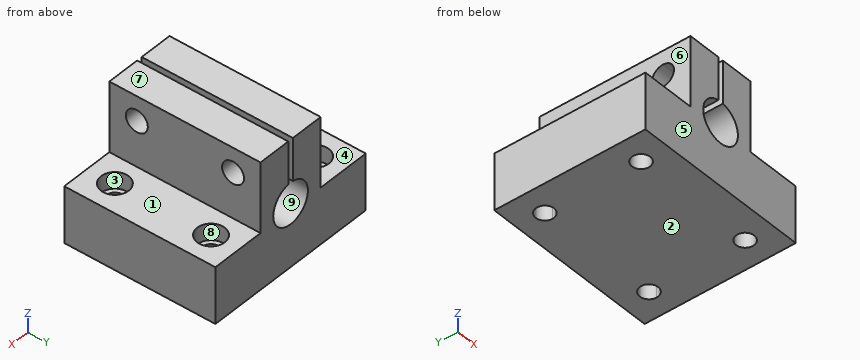
```python
from build123d import *

# Parameters (mm, degrees)
F0_W      = 65
F0_H      = 55
F1_DEPTH  = 20.5
F2_W      = 12
F2_H      = 55
F3_DEPTH  = 25.5
F5_DEPTH  = 74.8
F7_DEPTH  = 37.2
F9_R      = 5
F9_R_2    = 3.3
F10_DEPTH = 6
F8_R      = 3.3
F11_DEPTH = 45.5


with BuildPart() as f1:
    # F0 (on Top) → F1 (new body)
    with BuildSketch(Plane.XY):
        with Locations((32.5, 27.5)):
            Rectangle(F0_W, F0_H)
    extrude(amount=F1_DEPTH)

    # F2 (on face) → F3 (join)
    with BuildSketch(Plane.XY.offset(20.5)):
        with Locations((25.5, 27.5)):
            Rectangle(F2_W, F2_H)
        with Locations((39.5, 27.5)):
            Rectangle(F2_W, F2_H)
    extrude(amount=F3_DEPTH)

    # F4 (on face) → F5 (cut)
    with BuildSketch(Plane.XZ):
        with BuildLine():
            ThreePointArc((25, 23), (32.5, 15.5), (40, 23))
            ThreePointArc((40, 23), (32.5, 30.5), (25, 23))
        make_face()
    extrude(amount=-F5_DEPTH, mode=Mode.SUBTRACT)

    # F6 (on face) → F7 (cut)
    with BuildSketch(Plane(origin=(19.5, 0, 0), x_dir=(0, -1, 0), z_dir=(-1, 0, 0))):
        with BuildLine():
            ThreePointArc((-45, 41), (-47.8284271247, 34.1715728753), (-41, 37))
            ThreePointArc((-41, 37), (-42.1715728753, 39.8284271247), (-45, 41))
        make_face()
        with BuildLine():
            ThreePointArc((-10, 41), (-12.8284271247, 34.1715728753), (-6, 37))
            ThreePointArc((-6, 37), (-7.1715728753, 39.8284271247), (-10, 41))
        make_face()
    extrude(amount=-F7_DEPTH, mode=Mode.SUBTRACT)

    # F9 (on face) → F10 (cut)
    with BuildSketch(Plane.XY.offset(20.5)):
        with Locations((55, 45)):
            Circle(F9_R)
        with Locations((55, 45)):
            Circle(F9_R_2, mode=Mode.SUBTRACT)
        with BuildLine():
            ThreePointArc((15, 45), (10, 50), (5, 45))
            ThreePointArc((5, 45), (10, 40), (15, 45))
        make_face()
        with BuildLine():
            ThreePointArc((13.3, 45), (10, 41.7), (6.7, 45))
            ThreePointArc((6.7, 45), (10, 48.3), (13.3, 45))
        make_face(mode=Mode.SUBTRACT)
        with BuildLine():
            ThreePointArc((15, 10), (6.4644660941, 13.5355339059), (10, 5))
            ThreePointArc((10, 5), (13.5355339059, 6.4644660941), (15, 10))
        make_face()
        with BuildLine():
            ThreePointArc((13.3, 10), (12.3334523779, 7.6665476221), (10, 6.7))
            ThreePointArc((10, 6.7), (7.6665476221, 12.3334523779), (13.3, 10))
        make_face(mode=Mode.SUBTRACT)
        with Locations((55, 10)):
            Circle(F9_R)
        with Locations((55, 10)):
            Circle(F9_R_2, mode=Mode.SUBTRACT)
    extrude(amount=-F10_DEPTH, mode=Mode.SUBTRACT)

    # F8 (on face) → F11 (cut)
    with BuildSketch(Plane(origin=(0, 0, 0), x_dir=(1, 0, 0), z_dir=(0, 0, -1))):
        with BuildLine():
            ThreePointArc((13.3, -45), (7.6665476221, -42.6665476221), (10, -48.3))
            ThreePointArc((10, -48.3), (12.3334523779, -47.3334523779), (13.3, -45))
        make_face()
        with BuildLine():
            ThreePointArc((58.3, -45), (52.6665476221, -42.6665476221), (55, -48.3))
            ThreePointArc((55, -48.3), (57.3334523779, -47.3334523779), (58.3, -45))
        make_face()
        with Locations((55, -10)):
            Circle(F8_R)
        with BuildLine():
            ThreePointArc((13.3, -10), (10, -6.7), (6.7, -10))
            ThreePointArc((6.7, -10), (10, -13.3), (13.3, -10))
        make_face()
    extrude(amount=-F11_DEPTH, mode=Mode.SUBTRACT)


solid = f1.part
```
Read the model definition and answer for the solid it produces. Units are mm, in the model's axes. Face numbers are marked on the shaded views. A direction names the side the tool comes from. Give positions to 0.01 mm unless a question says otherwise; leave off trailing zeros. Order: outer loops, then holes, each group sorted by start corner. A loop starts at its lowest first (then second) coordinate and runs counter-clockwise, first axis right, second up.
(1) For a pull along X with two mould halves and no side action, classify the marked faces 6, 7, 8 and 9 as released by +X, released by -X, zero draft, split by the parting line, or undercut.
(2) Find section D-D (x = 32.5). Give the vertices of the cut face in (y, z), plus the area to 4 significant figures.
(3) Find section A-A (z = 13). Give the vertices of the cut face in (x, y), plus the area to 3 significant figures.
(4) For the marked faces 1, 2, 3, 4 and 5, determine the directions among +Z, -Z, +X, -X, +Y, -Y from which every point of the face is accessible in a straight line to the end or side of a thin tool.
(5) Find section B-B (y = 28.5). Give the vertices of the cut face in (x, z).
(6) Straight lines are drawn through the part: L1, parallel to Y at x = 55, z = 19; L2, parallel to Y at x = 10, z = 8; L3, parallel to X at y = 13.5, z = 44.5. For each, find the intervals that lie inside material, in ascending order.
(7) Find section C-C (z = 34). Give the vertices of the cut face in (x, y).
(8) Given pin 1 (12.5 mm diameter, centred on y = 36.5, z = 39, fed in from -X); pin 2 (6.5 mm diameter, centred on y = 10, z = 37, fed in from -X); pin 3 (13 mm diameter, centred on y = 38.5, z = 29.5, fed in from +X); pin 4 (11.5 mm diameter, centred on x = 10, y = 10, fed in from +Z), each flat-ended and moving along its own axis, determine where each tip first touches the part or whether it passes through.
Result sheet:
1. face 6: released by -X
1. face 7: zero draft
1. face 8: undercut
1. face 9: undercut
2. outline: (0, 0) - (55, 0) - (55, 15.5) - (0, 15.5) - close
2. area: 852.5 mm2
3. outline: (0, 0) - (65, 0) - (65, 55) - (0, 55) - close; hole circle Ø6.6 at (10, 10); hole circle Ø6.6 at (10, 45); hole circle Ø6.6 at (55, 10); hole circle Ø6.6 at (55, 45)
3. area: 3,440 mm2
4. face 1: +Z, +X, +Y, -Y
4. face 2: -Z, +X, -X, +Y, -Y
4. face 3: +Z
4. face 4: +Z, -X, +Y, -Y
4. face 5: +Z, -Z, +X, -X, -Y
5. outline: (0, 0) - (65, 0) - (65, 20.5) - (45.5, 20.5) - (45.5, 46) - (33.5, 46) - (33.5, 30.43) arc R7.5 cw (long way) to (31.5, 30.43) - (31.5, 46) - (19.5, 46) - (19.5, 20.5) - (0, 20.5) - close
6. L1: y = 0 to 5, 15 to 40, 50 to 55
6. L2: y = 0 to 6.7, 13.3 to 41.7, 48.3 to 55
6. L3: x = 19.5 to 31.5, 33.5 to 45.5
7. outline: (19.5, 0) - (31.5, 0) - (31.5, 7.35) - (19.5, 7.35) - close; (19.5, 12.65) - (31.5, 12.65) - (31.5, 42.35) - (19.5, 42.35) - close; (19.5, 47.65) - (31.5, 47.65) - (31.5, 55) - (19.5, 55) - close; (33.5, 0) - (45.5, 0) - (45.5, 7.35) - (33.5, 7.35) - close; (33.5, 12.65) - (45.5, 12.65) - (45.5, 42.35) - (33.5, 42.35) - close; (33.5, 47.65) - (45.5, 47.65) - (45.5, 55) - (33.5, 55) - close
8. pin 1: stops at x = 19.5
8. pin 2: passes through
8. pin 3: stops at x = 45.5
8. pin 4: stops at z = 20.5
